For this review, take the finished solid that the model builds, in its own axes (mm). Face numbers are marked on the shaded views. Coordinates: 2 decimals unless noted, no trailing zeros. Order: outer loops, then holes, each group sorted by start corner. A loop starts at its lowest first (then second) coordinate and runs counter-clockwise, first axis right, second up. Notation, with made-up numbers: (35.25, 26) - (57.25, 26) arc R17 cw to (57.25, 50) - close; hole circle Ø8 at (-32, -33.5). An arc over 180 degrees is marked (long way). One line per item, written item: value. Start each with the question number.
(1) To check wall thickness, follow line 1 along Y through (x, z) = (-5.5, 34); line 2 along X through (y, z) = (11, 4); line 3 along Z through (x, y) = (1, 29.5). State the ranges of each line that lie inside material, in increasing order.
(2) Consider section A-A on z = 10. Write out the cut boundary in (x, y).
(3) Consider section D-D on y = -1. Write out the cut boundary in (x, z), then the cut area to 3 significant figures.
(4) Mouldability with a two-part tool opening along Y and no side actions: class the marked faces 1, 2, 3 and 4 as released by +Y, released by -Y, zero draft, split by the parting line, or undercut.
(5) Consider section B-B on x = -11.5. Write out the cut boundary in (y, z).
(6) Clearance check with flat-ended pins moving along their axes: pin 1 (4 mm diameter, centred on x = -8, z = 15, fed in from -Y); pin 2 (0.9 mm diameter, centred on x = 18, y = 7, fed in from +Z). State where each tip first meets the part, or that it passes through.
(7) Consider section C-C on z = 25. Write out the cut boundary in (x, y), then the cut area to 3 significant figures.
Autodesk Inventor part; units mm, degrees
ref_plane "YZ Plane" through (0, 0, 0) normal (1, 0, 0) x (0, 1, 0)
ref_plane "XZ Plane" through (0, 0, 0) normal (0, 1, 0) x (-1, 0, 0)
ref_plane "XY Plane" through (0, 0, 0) normal (0, 0, 1) x (1, 0, 0)
sketch "스케치1" plane through (0, 0, 0) normal (0, 0, 1) x (1, 0, 0)
  line L0 (-16.7, 28.2) -> (16.7, 28.2)
  line L1 (16.7, 28.2) -> (16.7, -28.2)
  line L2 (16.7, -28.2) -> (-16.7, -28.2)
  line L3 (-16.7, -28.2) -> (-16.7, 28.2)
  line L4 (19.7, -31.2) -> (19.7, 31.2)
  line L5 (19.7, 31.2) -> (-19.7, 31.2)
  line L6 (-19.7, 31.2) -> (-19.7, -31.2)
  line L7 (-19.7, -31.2) -> (19.7, -31.2)
  point P0 (0, 0)
  point P1 (-16.7, 0)
  point P2 (0, 28.2)
  dimension "d0" = 33.4
  dimension "d1" = 56.4
  dimension "d2" = 3
extrude "돌출1" add sketch "스케치1" along normal blind 5
sketch "스케치3" plane through (-19.7, -31.2, 0) normal (0, -1, 0) x (1, 0, 0)
  line L0 (39.4, 0) -> (0, 0)
  line L1 (0, 0) -> (39.4, 0)
  line L2 (39.4, 0) -> (39.4, 39)
  line L3 (39.4, 39) -> (0, 39)
  line L4 (0, 39) -> (0, 0)
  line L5 (19.7, 39) -> (19.7, 0) construction
  line L6 (0, 36) -> (39.4, 36) construction
  circle A0 centre (19.7, 36) radius 11 construction
  circle A1 centre (8.7, 36) radius 1.3
  circle A2 centre (11.9218, 28.2218) radius 1.3
  circle A3 centre (19.7, 25) radius 1.3
  circle A4 centre (27.4782, 28.2218) radius 1.3
  circle A5 centre (30.7, 36) radius 1.3
  line L7 (0, 15) -> (39.4, 15) construction
  circle A6 centre (11.7, 15) radius 1.3
  circle A7 centre (27.7, 15) radius 1.3
  point P0 (39.4, 0)
  dimension "d9" = 22
  dimension "d5" = 39
  dimension "d8" = 3
  dimension "d10" = 2.6
  dimension "d13" = 180
  dimension "d15" = 24
  dimension "d16" = 2.6
  dimension "d17" = 2.6
  dimension "d18" = 8
  dimension "d19" = 8
extrude "돌출2" add sketch "스케치3" against normal blind 3
mirror "미러1" about plane through (0, 0, 0) normal (0, 1, 0)
properties part number "ARM_1 SKETCH"
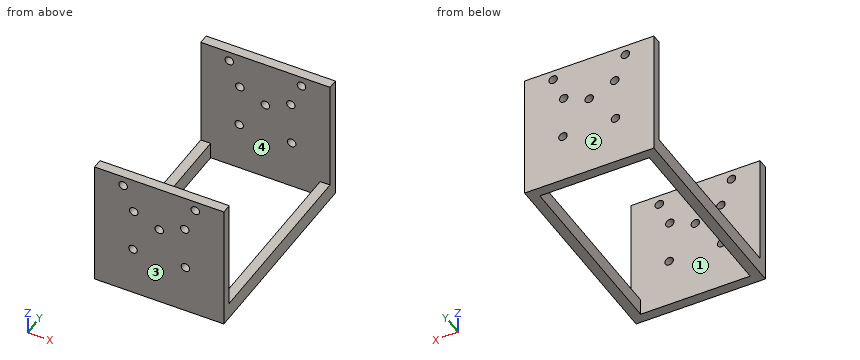
Geometry check:
1. line 1: y = -31.2 to -28.2, 28.2 to 31.2
1. line 2: x = -19.7 to -16.7, 16.7 to 19.7
1. line 3: z = 0 to 24.17, 25.83 to 39
2. outline: (-19.7, -31.2) - (19.7, -31.2) - (19.7, -28.2) - (-19.7, -28.2) - close; (-19.7, 28.2) - (19.7, 28.2) - (19.7, 31.2) - (-19.7, 31.2) - close
3. outline: (-19.7, 0) - (-16.7, 0) - (-16.7, 5) - (-19.7, 5) - close; (16.7, 0) - (19.7, 0) - (19.7, 5) - (16.7, 5) - close
3. area: 30.0 mm^2
4. face 1: undercut
4. face 2: released by +Y
4. face 3: released by -Y
4. face 4: undercut
5. outline: (-31.2, 0) - (-28.2, 0) - (-28.2, 34.8) - (-31.2, 34.8) - close; (-31.2, 37.2) - (-28.2, 37.2) - (-28.2, 39) - (-31.2, 39) - close; (28.2, 0) - (31.2, 0) - (31.2, 34.8) - (28.2, 34.8) - close; (28.2, 37.2) - (31.2, 37.2) - (31.2, 39) - (28.2, 39) - close
6. pin 1: stops at y = -31.2
6. pin 2: stops at z = 5
7. outline: (-19.7, -31.2) - (-1.3, -31.2) - (-1.3, -28.2) - (-19.7, -28.2) - close; (-19.7, 28.2) - (-1.3, 28.2) - (-1.3, 31.2) - (-19.7, 31.2) - close; (1.3, -31.2) - (19.7, -31.2) - (19.7, -28.2) - (1.3, -28.2) - close; (1.3, 28.2) - (19.7, 28.2) - (19.7, 31.2) - (1.3, 31.2) - close
7. area: 221 mm^2
